from build123d import *

# Parameters (mm, degrees)
SKETCH1_R               = 1.7499999999999998
SKETCH1_R_2             = 9
MOTOR_PLATE_DEPTH       = 5
BOSS_EXTRUDE1_DEPTH     = 35
BOSS_EXTRUDE2_START     = 35
BOSS_EXTRUDE2_DEPTH     = 35
CUT_EXTRUDE5_DEPTH      = 100.75732766200707
CUT_EXTRUDE5_DEPTH_BACK = 100.75732766200707
SKETCH11_R              = 2.7500000000000084
SKETCH11_R_2            = 2.750000000000008
CUT_EXTRUDE7_DEPTH      = 100.75732766200707
CUT_EXTRUDE7_DEPTH_BACK = 100.75732766200707
SKETCH14_W              = 20.499999999999986
SKETCH14_H              = 5
FILLET4_R               = 5
BOSS_EXTRUDE5_DEPTH     = 7.5
CUT_EXTRUDE14_DEPTH     = 98.1044493253111
SKETCH27_R              = 2.3500000000000005
CUT_EXTRUDE15_DEPTH     = 4
SKETCH28_R              = 1.7499999999999998
SKETCH28_R_2            = 1.7500000000000004
CUT_EXTRUDE16_DEPTH     = 7
FILLET5_R               = 2.5
FILLET6_R               = 10


with BuildPart() as part:
    # Sketch1 → Motor Plate (new body)
    with BuildSketch(Plane(origin=(0, 0, 0), x_dir=(1, 0, 0), z_dir=(0, 1, 0))):
        with BuildLine():
            Line((-24.237109976232734, 15.250000000000002), (-85.24999999999999, 15.25))
            Line((-85.24999999999999, 15.25), (-85.24999999999999, 10.25))
            Line((-85.24999999999999, 10.25), (-64.75, 10.25))
            Line((-64.75, 10.25), (-64.75, -10.250000000000002))
            Line((-64.75, -10.250000000000002), (-85.24999999999999, -10.250000000000002))
            Line((-85.24999999999999, -10.250000000000002), (-85.24999999999999, -15.250000000000002))
            Line((-85.24999999999999, -15.250000000000002), (-24.237109976232734, -15.25))
            ThreePointArc((-24.237109976232734, -15.25), (-20.505009839771837, -15.972531133362475), (-17.31222141159481, -18.03571428571429))
            ThreePointArc((-17.31222141159481, -18.03571428571429), (-14.020240375434447, -20.698619756279353), (-10.326086956521745, -22.76778268005806))
            ThreePointArc((-10.326086956521745, -22.76778268005806), (-8.416527322228076, -22.627457016016997), (-7.500000000000001, -20.94636006565341))
            Line((-7.500000000000001, -20.94636006565341), (-7.500000000000001, -15))
            ThreePointArc((-7.500000000000001, -15), (-6.914213562373096, -13.585786437626904), (-5.500000000000001, -13))
            Line((-5.500000000000001, -13), (5.499999999999999, -13))
            ThreePointArc((5.499999999999999, -13), (6.914213562373094, -13.585786437626904), (7.499999999999999, -15))
            Line((7.499999999999999, -15), (7.499999999999999, -20.94636006565341))
            ThreePointArc((7.499999999999999, -20.94636006565341), (8.416527322228072, -22.627457016016997), (10.32608695652174, -22.76778268005806))
            ThreePointArc((10.32608695652174, -22.76778268005806), (20.698619756279356, 14.020240375434444), (-17.31222141159481, 18.035714285714285))
            ThreePointArc((-17.31222141159481, 18.035714285714285), (-20.50500983977184, 15.972531133362477), (-24.237109976232734, 15.250000000000002))
        make_face()
        with Locations(Location((8.838834764831846, 8.838834764831835, 0), (0, 0, 270))):
            Circle(SKETCH1_R, mode=Mode.SUBTRACT)
        with Locations(Location((-8.838834764831843, 8.838834764831846, 0), (0, 0, 270))):
            Circle(SKETCH1_R, mode=Mode.SUBTRACT)
        with Locations(Location((-8.838834764831843, -8.838834764831846, 0), (0, 0, 270))):
            Circle(SKETCH1_R, mode=Mode.SUBTRACT)
        with Locations(Location((8.838834764831846, -8.838834764831835, 0), (0, 0, 270))):
            Circle(SKETCH1_R, mode=Mode.SUBTRACT)
        with Locations(Location((0, 0, 0), (0, 0, 270))):
            Circle(SKETCH1_R_2, mode=Mode.SUBTRACT)
    extrude(amount=MOTOR_PLATE_DEPTH)

    # Sketch3 → Boss-Extrude1 (add)
    with BuildSketch(Plane.XZ):
        Polygon((-85.24999999999999, 15.250000000000002), (-85.24999999999999, 10.250000000000002), (-64.75, 10.250000000000002), (-64.75, -10.25), (-85.24999999999999, -10.25), (-85.24999999999999, -15.25), (-59.75, -15.25), (-59.75, 15.250000000000002), align=None)
    extrude(amount=BOSS_EXTRUDE1_DEPTH)

    # Sketch4 → Boss-Extrude2 (add)
    with BuildSketch(Plane.XZ.offset(BOSS_EXTRUDE2_START)):
        with BuildLine():
            Line((-59.75, -15.25), (-59.75, 15.250000000000002))
            Line((-59.75, 15.250000000000002), (-24.237109976232734, 15.25))
            ThreePointArc((-24.237109976232734, 15.25), (-23.15840811564324, 15.30835012203906), (-22.09229473209558, 15.482719540807848))
            ThreePointArc((-22.09229473209558, 15.482719540807848), (-21.052891601024875, 15.071238646911935), (-21.04437270453208, 13.953382295083351))
            ThreePointArc((-21.04437270453208, 13.953382295083351), (-25.250000000000007, 3.09e-15), (-21.044372704532076, -13.953382295083353))
            ThreePointArc((-21.044372704532076, -13.953382295083353), (-21.05289160102487, -15.071238646911937), (-22.092294732095578, -15.48271954080785))
            ThreePointArc((-22.092294732095578, -15.48271954080785), (-23.15840811564324, -15.308350122039062), (-24.237109976232734, -15.25))
            Line((-24.237109976232734, -15.25), (-59.75, -15.25))
        make_face()
    extrude(amount=-BOSS_EXTRUDE2_DEPTH)

    # Sketch11 → Cut-Extrude5 (cut, two sides: drawn at the far end of the back side and taken through both)
    with BuildSketch(Plane(origin=(-4.3e-16, 0, -15.250000000000002), x_dir=(-1, 0, 6e-17), z_dir=(-6e-17, 0, -1)).offset(-CUT_EXTRUDE5_DEPTH_BACK)):
        with Locations((75, -25)):
            Circle(SKETCH11_R)
        with Locations((75, -5.000000000000001)):
            Circle(SKETCH11_R_2)
    extrude(amount=CUT_EXTRUDE5_DEPTH + CUT_EXTRUDE5_DEPTH_BACK, mode=Mode.SUBTRACT)

    # Sketch14 → Cut-Extrude7 (cut, two sides: drawn at the far end of the back side and taken through both)
    with BuildSketch(Plane(origin=(-4.3e-16, 0, -15.250000000000002), x_dir=(-1, 0, 6e-17), z_dir=(-6e-17, 0, -1)).offset(-CUT_EXTRUDE7_DEPTH_BACK)):
        with Locations((75, 2.5)):
            Rectangle(SKETCH14_W, SKETCH14_H)
    extrude(amount=CUT_EXTRUDE7_DEPTH + CUT_EXTRUDE7_DEPTH_BACK, mode=Mode.SUBTRACT)

    # Fillet4
    fillet4_edges = [part.edges().sort_by_distance(p)[0] for p in [
        (-85.24999999999999, 0, -12.75),
        (-85.24999999999999, 0, 12.75),
        (-85.24999999999999, -35, -12.75),
        (-85.24999999999999, -35, 12.750000000000002),
    ]]
    fillet(fillet4_edges, radius=FILLET4_R)

    # Sketch24 → Boss-Extrude5 (add)
    with BuildSketch(Plane(origin=(0, -29.8908, 0), x_dir=(-1, 0, 0), z_dir=(0, -1, 0))):
        with BuildLine():
            Line((24.237109976232734, 15.25), (28.819440187957916, 15.25))
            Line((28.819440187957916, 15.25), (13.970450097258862, 30.09899009069905))
            ThreePointArc((13.970450097258862, 30.09899009069905), (12.44663498380185, 30.730174977242044), (10.92281987034484, 30.09899009069905))
            Line((10.92281987034484, 30.09899009069905), (8.062504135197518, 27.238674355551726))
            Line((8.062504135197518, 27.238674355551726), (8.165668965896261, 23.893186274320946))
            ThreePointArc((8.165668965896261, 23.893186274320946), (15.42746120991581, 19.988895432628166), (21.044372704532083, 13.95338229508334))
            ThreePointArc((21.044372704532083, 13.95338229508334), (21.052891601024868, 15.07123864691193), (22.092294732095578, 15.482719540807848))
            ThreePointArc((22.092294732095578, 15.482719540807848), (23.15840811564324, 15.30835012203906), (24.237109976232734, 15.25))
        make_face()
    extrude(amount=-BOSS_EXTRUDE5_DEPTH)

    # Sketch26 → Cut-Extrude14 (cut, through all)
    with BuildSketch(Plane.XZ.offset(29.8908)):
        with BuildLine():
            Line((-18.976555851670547, -8.317283119898706), (-13.970450097258862, -30.09899009069905))
            Line((-13.970450097258862, -30.09899009069905), (-30.098990090699047, -13.970450097258864))
            ThreePointArc((-30.098990090699047, -13.970450097258864), (-30.730174977242033, -12.446634983801854), (-30.098990090699044, -10.92281987034485))
            Line((-30.098990090699044, -10.92281987034485), (-27.238674355551726, -8.062504135197523))
            Line((-27.238674355551726, -8.062504135197523), (-18.976555851670547, -8.317283119898706))
        make_face()
    extrude(amount=CUT_EXTRUDE14_DEPTH, mode=Mode.SUBTRACT)

    # Sketch27 → Cut-Extrude15 (cut)
    with BuildSketch(Plane.XZ.offset(29.8908)):
        with Locations(Location((-27.29099835192915, -12.473575752165065, 0), (0, 0, 270))):
            Circle(SKETCH27_R)
        with Locations(Location((-12.47357575216505, -27.290998351929158, 0), (0, 0, 270))):
            Circle(SKETCH27_R)
    extrude(amount=-CUT_EXTRUDE15_DEPTH, mode=Mode.SUBTRACT)

    # Sketch28 → Cut-Extrude16 (cut)
    with BuildSketch(Plane.XZ.offset(29.8908)):
        with Locations(Location((-27.29099835192915, -12.473575752165065, 0), (0, 0, 270))):
            Circle(SKETCH28_R)
        with Locations(Location((-12.47357575216505, -27.290998351929158, 0), (0, 0, 270))):
            Circle(SKETCH28_R_2)
    extrude(amount=-CUT_EXTRUDE16_DEPTH, mode=Mode.SUBTRACT)

    # Fillet5
    # the kernel refuses this fillet: 2.5 mm, written as the material it takes off along each edge
    with BuildSketch(Plane(origin=(-8.165668965896261, -34.068034873717735, -23.89318627432096), x_dir=(-0.9355866460023518, 0, 0.35309719316651356), z_dir=(0, 1, 0))) as fillet5_piece_1:
        with BuildLine():
            CenterArc((1.6727559192968875, -2.498754534741212), FILLET5_R, 91.80863723012877, 65.74822155289536)
            Line((-0.6378911862633408, -1.54433850723217), (0, 0))
            ThreePointArc((0, 0), (0.7969261690989898, -0.0125791991137666), (1.59385233819798, 7e-17))
        make_face()
    extrude(amount=15.854469747435477, mode=Mode.SUBTRACT)
    with BuildSketch(Plane(origin=(-28.819440187957913, -29.8908, -15.249999999999998), x_dir=(-0.5820598075620075, 0, 0.8131459773133474), z_dir=(0, -1, 0))) as fillet5_piece_2:
        with BuildLine():
            CenterArc((4.594416541128744, 2.123375145412493), FILLET5_R, 144.40445067780377, 93.73659766899215)
            Line((2.5615515978453756, 3.578524664317512), (2.3582651035170388, 3.724039616208014))
            Line((2.3582651035170388, 3.724039616208014), (-0.20328649432833684, 0.14551495189050187))
            Line((-0.20328649432833684, 0.14551495189050187), (0.0408506494173984, -0.24663986790901668))
            ThreePointArc((0.0408506494173984, -0.24663986790901668), (1.826086075758527, 0.04904641812113162), (3.142884119812632, -0.21233751454124886))
            Line((3.142884119812632, -0.21233751454124886), (3.274841612659551, 3e-17))
        make_face()
    extrude(amount=16.111297914021037, mode=Mode.SUBTRACT)
    with BuildSketch(Plane(origin=(-23.893186274320946, -29.8908, -8.16566896589627), x_dir=(-0.2624644085594799, 0, 0.9649416740091198), z_dir=(0, -1, 0))) as fillet5_piece_3:
        with BuildLine():
            CenterArc((3.375802522576318, 2.494923627384301), FILLET5_R, 163.59172174149506, 102.75638657572608)
            Line((0.977619595016342, 3.2011237732069016), (0, 0))
            ThreePointArc((0, 0), (1.6082832772651305, 0.05127136341856297), (3.216566554530266, 6e-17))
        make_face()
    extrude(amount=13.476895876087362, mode=Mode.SUBTRACT)

    # Fillet6
    fillet6_edges = [part.edges().sort_by_distance(p)[0] for p in [
        (-28.819440187957916, -26.1408, -15.25),
    ]]
    fillet(fillet6_edges, radius=FILLET6_R)


solid = part.part
For this review, take the finished solid that the model builds, in its own axes (mm). A direction names the side the tool comes from. Give positions to 0.01 mm unless a question says otherwise; leave off trailing zeros. Order: outer loops, then holes, each group sorted by start corner. A loop starts at its lowest first (then second) coordinate and runs counter-clockwise, first axis right, second up. Notation, with made-up numbers: M 59,88.25 L 78,88.25 A13 ccw 78,100.25 Z; hole C 56,17.5 d4. An arc over 180 degrees is marked long. Answer in a Markdown table with one row per item. Add a question column.
(1) Consider section B-B on x = 0. State the section outline as (y, z) points, and give its area (3 significant figures).
(2) Consider section D-D on y = -3.5. State the section outline as (x, z) points, and give its area (3 significant figures).
(3) Consider section C-C on z = 0. State the section outline as (x, y) points.
(4) Consider section A-A on x = -75. State the section outline as (y, z) points.
(5) Mouldability with a two-part tool opening along X and no side actions: class faces 6 (the face through (-25.556, -24.412, -12.246)), 7 (the face through (-28.689, -32.41, -9.513)), 8 (the face through (-85.25, -17, -13)), 9 (the face through (-75, -17, -10.25)) as +X half, -X half, draft (parallel to the pull), parting line (faces both ways), or undercut.
(6) For faces 1 (the face through (-20, -29.891, -19)), 2 (the face through (-75, -17, 10.25)), 3 (the face through (-55, -15, 15.25)), 4 (the face through (-72, 0, 13)), 5 (the face through (-7.5, 2, 18)), list the 3-axis set-ups (+Z, -Z, +X, -X, +Y, -Y) from which the entire face can be reached by the end or side of a thin tool; tool diameter is ignored.
(7) For pin 1 (4 mm diameter, centred on x = -12.5, z = -26.5, fed in from -Y); pin 2 (4.5 mm diameter, centred on x = 8.84, z = -8.84, fed in from -Y); pin 3 (9 mm diameter, centred on x = -75, y = -25, fed in from -Z), all flat-tipped, find the tip position at first contact; note any pin that passes through.
(8) Wall thickness on probe 1 along Z at (x, y) = (-79.5, -30.5); probe 2 along X at (y, z) = (4, 0): over which ranges is each line inside the solid? List them lowest first. Write a range as [from, to].
Evaluation:
| question | item | result |
|---|---|---|
| 1 | outline | M 0,-25 L 5,-25 L 5,-9 L 0,-9 Z; M 0,9 L 5,9 L 5,13 L 0,13 Z |
| 1 | area | 100 mm^2 |
| 2 | outline | M -85.02,-15.25 L -77.3,-15.25 L -77.3,-10.25 L -85.02,-10.25 Z; M -85.02,10.25 L -77.3,10.25 L -77.3,15.25 L -85.02,15.25 Z; M -72.7,-15.25 L -24.24,-15.25 A10 cw -22.09,-15.48 A1 ccw -21.04,-13.95 A25.25 cw -21.04,13.95 A1 ccw -22.09,15.48 A10 cw -24.24,15.25 L -72.7,15.25 L -72.7,10.25 L -64.75,10.25 L -64.75,-10.25 L -72.7,-10.25 Z |
| 2 | area | 1,410 mm^2 |
| 3 | outline | M -64.75,-35 L -25.25,-35 L -25.25,0 L -9,0 L -9,5 L -64.75,5 Z; M 9,0 L 25,0 L 25,5 L 9,5 Z |
| 4 | outline | M -35,-15.25 L -27.75,-15.25 L -27.75,-10.25 L -35,-10.25 Z; M -35,10.25 L -27.75,10.25 L -27.75,15.25 L -35,15.25 Z; M -22.25,-15.25 L -7.75,-15.25 L -7.75,-10.25 L -22.25,-10.25 Z; M -22.25,10.25 L -7.75,10.25 L -7.75,15.25 L -22.25,15.25 Z; M -2.25,-15.25 L 0,-15.25 L 0,-10.25 L -2.25,-10.25 Z; M -2.25,10.25 L 0,10.25 L 0,15.25 L -2.25,15.25 Z |
| 5 | face 6 | undercut |
| 5 | face 7 | +X half |
| 5 | face 8 | -X half |
| 5 | face 9 | draft |
| 6 | face 1 | -Z, +X, -Y |
| 6 | face 2 | -X, +Y, -Y |
| 6 | face 3 | +Z, -X, +Y, -Y |
| 6 | face 4 | +Z, -Z, -X, +Y |
| 6 | face 5 | +Z, +Y, -Y |
| 7 | pin 1 | stops at y = -29.89 |
| 7 | pin 2 | stops at y = 0 |
| 7 | pin 3 | stops at z = -15.25 |
| 8 | probe 1 | z = [-15.25, -10.25], [10.25, 15.25] |
| 8 | probe 2 | x = [-64.75, -9], [9, 25] |
